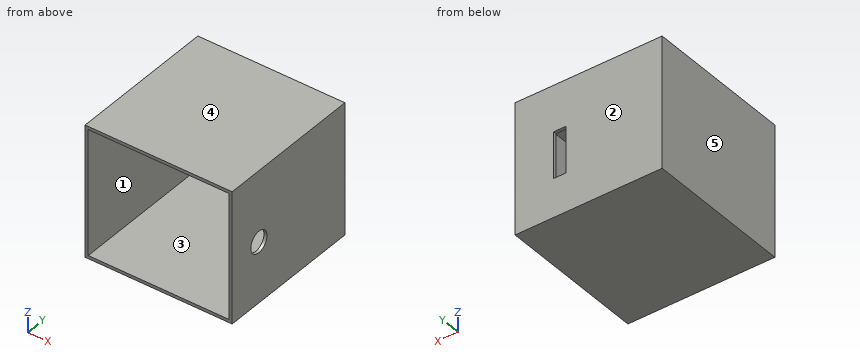
```python
from build123d import *

# Parameters (mm, degrees)
F0_W      = 95
F0_H      = 96.059554
F1_DEPTH  = 85
F2_T      = -2
F3_R      = 6.924471
F4_DEPTH  = 65.166272
F4_FACE_R = 6.924471
F5_DEPTH  = 140.461847
F6_W      = 8
F6_H      = 30
F7_DEPTH  = 21.398656


with BuildPart() as f1:
    # F0 (on Top) → F1 (new body)
    with BuildSketch(Plane.XY):
        with Locations((-47.5, -48.029777)):
            Rectangle(F0_W, F0_H)
    extrude(amount=F1_DEPTH)

    # F2
    f2_openings = [f1.faces().sort_by_distance(p)[0] for p in [
        (-47.5, -96.059554, 42.5),
    ]]
    offset(amount=F2_T, openings=f2_openings)

    # F3 (on face) → F4 (join)
    with BuildSketch(Plane.YZ):
        with Locations((-73.268585, 39.188489)):
            Circle(F3_R)
    extrude(amount=-F4_DEPTH)

    # F4_face (on face) → F5 (cut)
    with BuildSketch(Plane(origin=(-65.166272, -73.268585, 39.188489), x_dir=(0, 1, 0), z_dir=(-1, 0, 0))):
        Circle(F4_FACE_R)
    extrude(amount=-F5_DEPTH, mode=Mode.SUBTRACT)

    # F6 (on face) → F7 (cut)
    with BuildSketch(Plane(origin=(0, 0, 0), x_dir=(-1, 0, 0), z_dir=(0, 1, 0))):
        with Locations((28.885877, 40.065341)):
            Rectangle(F6_W, F6_H)
    extrude(amount=-F7_DEPTH, mode=Mode.SUBTRACT)


solid = f1.part
```
Design review of the part built by this model. Coordinates are the model's own, in mm. Face numbers are marked on the shaded views. A direction names the side the tool comes from. Give positions to 0.01 mm unless a question says otherwise; leave off trailing zeros. Write each loop counter-clockwise with the first axis right and the second up, starting at its lowest first coordinate (ties: lowest second). Pieces come first, ordered by that corner, then holes. Notation, with made-up numbers: (-31.5, 27) -> (-11.5, 27) arc R16 ccw to (-11.5, 37) -> close; hole circle Ø1 at (18.5, 12). An arc over 180 degrees is marked (long way). Answer in a Markdown table with one row per item.
(1) For the marked faces 1 and 2, list the 3-axis set-ups (+Z, -Z, +X, -X, +Y, -Y) from which the entire face can be reached by the end or side of a thin tool; tool diameter is ignored.
Results:
| item | result |
|---|---|
| face 1 | -Y |
| face 2 | +Z, -Z, +X, -X, +Y |
(2) Clearance check with a flat-ended pin moving along its axis: pin 1 (1 mm diameter, centred on x = -64.5, z = 70, fed in from -Y). State where the tip first meets the part, or that it passes through.
Results:
| item | result |
|---|---|
| pin 1 | y = -2 |
(3) Consider section A-A (z = 28.5). State the section outline as (x, y) points, then the cut area to 3 significant figures.
Results:
| item | result |
|---|---|
| outline | (-95, -96.06) -> (-93, -96.06) -> (-93, -2) -> (-32.89, -2) -> (-32.89, 0) -> (-95, 0) -> close; (-24.89, -2) -> (-2, -2) -> (-2, -96.06) -> (0, -96.06) -> (0, 0) -> (-24.89, 0) -> close |
| area | 550 mm2 |
(4) To check wall thickness, follow probe 1 along Z at (x, y) = (-73, -83); probe 2 along X at (y, z) = (-62, 8); probe 3 along Y at (x, z) = (-55.5, 28.5). State the ranges of each line that lie inside material, in increasing order.
Results:
| item | result |
|---|---|
| probe 1 | 0 to 2, 83 to 85 |
| probe 2 | -95 to -93, -2 to 0 |
| probe 3 | -2 to 0 |
(5) Consider section D-D (x = -84). State the section outline as (y, z) points, then the cut area to 3 significant figures.
Results:
| item | result |
|---|---|
| outline | (-96.06, 0) -> (0, 0) -> (0, 85) -> (-96.06, 85) -> (-96.06, 83) -> (-2, 83) -> (-2, 2) -> (-96.06, 2) -> close |
| area | 546 mm2 |
(6) Consider section B-B (y = -39). State the section outline as (x, z) points.
Results:
| item | result |
|---|---|
| outline | (-95, 0) -> (0, 0) -> (0, 85) -> (-95, 85) -> close; hole (-93, 2) -> (-2, 2) -> (-2, 83) -> (-93, 83) -> close |
(7) Mouldability with a two-part tool opening along Z and no side actions: class the marked faces 3, 4 and 5 as +Z half, -Z half, draft (parallel to the pull), parting line (faces both ways), or undercut.
Results:
| item | result |
|---|---|
| face 3 | undercut |
| face 4 | +Z half |
| face 5 | draft |
(8) Consider section C-C (z = 37.5). State the section outline as (x, y) points, then the cut area to 3 significant figures.
Results:
| item | result |
|---|---|
| outline | (-95, -96.06) -> (-93, -96.06) -> (-93, -2) -> (-32.89, -2) -> (-32.89, 0) -> (-95, 0) -> close; (-24.89, -2) -> (-2, -2) -> (-2, -66.55) -> (0, -66.55) -> (0, 0) -> (-24.89, 0) -> close; (-2, -96.06) -> (0, -96.06) -> (0, -79.98) -> (-2, -79.98) -> close |
| area | 523 mm2 |
